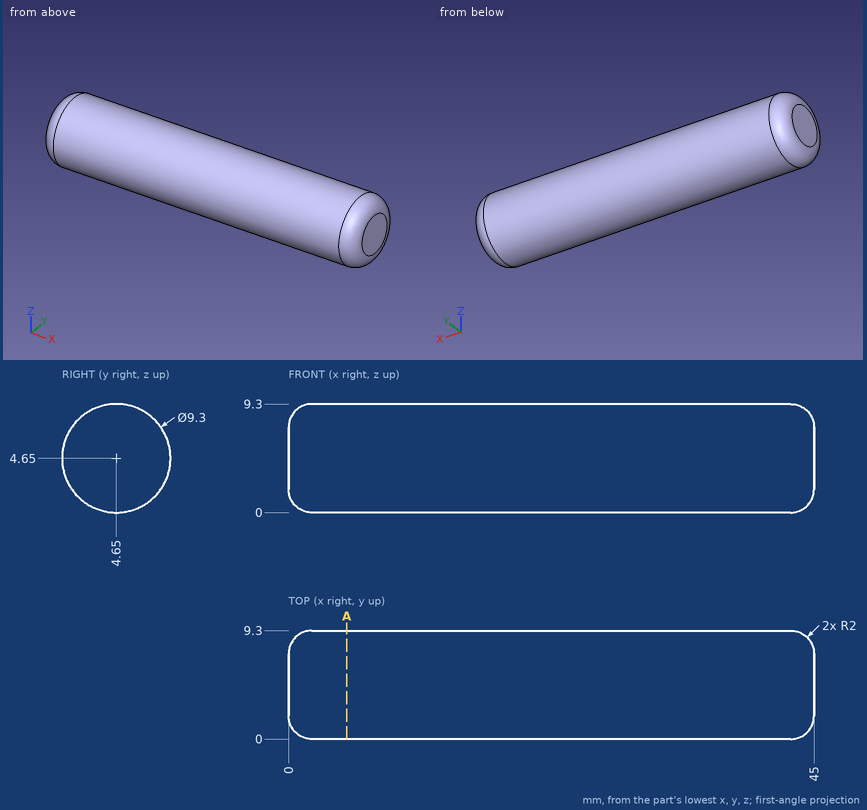
Geometry check sheet. Reference: drawing and pictorial views, mm from the part's lowest x, y, z. Coordinates: 2 decimals unless noted, no trailing zeros. Loops run counter-clockwise (first coordinate to the right, second up) from the corner with the lowest first, then second, coordinate; pieces in that order, holes last. Notation, with made-up numbers: (83.25, -36.5) -> (127.25, -36.5) arc R10 cw to (127.25, -21.5) -> close; hole circle Ø10 at (-40, 76.5). An arc over 180 degrees is marked (long way). Put each result on its own line as item: value.
1) Thickness scan on line 1 (Z direction, x = 31.5, y = 4.5); line 2 (X direction, y = 4, z = 2). Record the ranges inside material, lowest first.
Result set:
line 1: z = 0 to 9.3
line 2: x = 0 to 45
2) Cross-section at A-A on x = 5. Record the boundary of the cut face in (y, z).
Result set:
outline: circle Ø9.3 at (4.65, 4.65)
3) Gauge pin test, flat ends, axial feed: pin 1 Ø2 at (x, z) = (19, 3) entering from +Y; pin 2 Ø3 at (x, y) = (8, 5) entering from +Z; pin 3 Ø3 at (x, z) = (18.5, 2) entering from +Y; pin 4 Ø1 at (x, y) = (8, 1.5) entering from -Z. Record the tip position at first contact, or that the pin passes through.
Result set:
pin 1: stops at y = 9.25
pin 2: stops at z = 9.3
pin 3: stops at y = 9.16
pin 4: stops at z = 0.83
